Answer from the drawing. Dimensions are ordinates in mm from the lowest x, y and z of the part. A direction names the side the tool comes from. Give positions to 0.01 mm unless a question says otherwise; leave off trailing zeros.
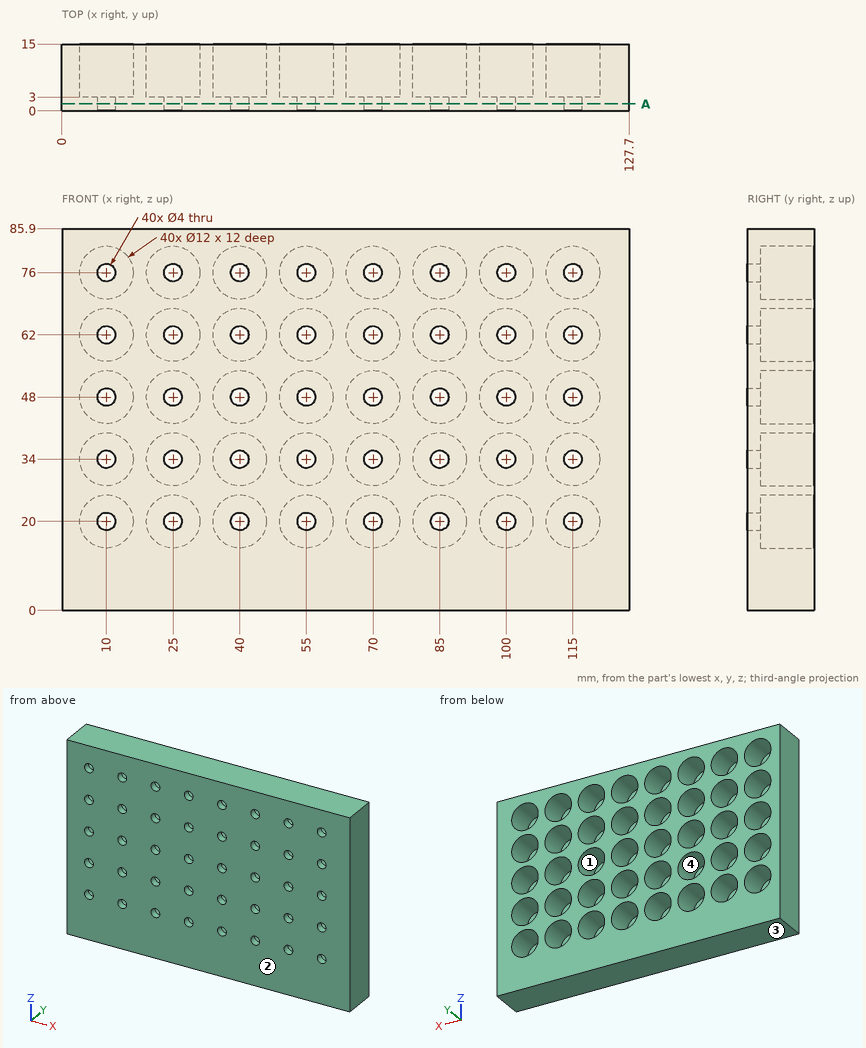
Item 1: Which of the six approach directions +Z, -Z, +X, -X, +Y, -Y give full straight-line access (tool end or side, diameter ignored) to the marked faces 1 and 2?
Conclusion:
face 1: +Y
face 2: +Z, -Z, +X, -X, -Y
Item 2: A cutting plane is placed at A-A, the plane y = 1.5. Count the separate pieces of the cut face and the enclosed holes in it, plus the area to 3 significant figures.
Conclusion:
separate pieces: 1
enclosed holes: 40
area: 10,500 mm2
Item 3: This flat-tipped pin is pushed along its axis until it touches: P1, Ø9.5, axis at x = 10, z = 48, coming from the +Y side. Where does it stop, or does it pass through?
Conclusion:
P1: stops at y = 3
Item 4: Consider probe 1 along Z at (x, y) = (100, 1.5); probe 2 along Z at (x, y) = (10, 9.5); probe 3 along Y at (x, z) = (28, 72). Determine where each line is inside the solid, lowest interval first.
Conclusion:
probe 1: z = 0 to 18, 22 to 32, 36 to 46, 50 to 60, 64 to 74, 78 to 85.9
probe 2: z = 0 to 14, 26 to 28, 40 to 42, 54 to 56, 68 to 70, 82 to 85.9
probe 3: y = 0 to 3
Item 5: Determine the mould class of the marked faces 3 and 4 for opening direction X: pulls with the +X half, pulls with the -X half, needs draft (parallel to the pull), parting line crosses it, or undercut.
Conclusion:
face 3: needs draft
face 4: undercut
